Verification items for the finished model (mm, model axes). Give positions to 0.01 mm unless a question says otherwise; leave off trailing zeros. Order: outer loops, then holes, each group sorted by start corner. A loop starts at its lowest first (then second) coordinate and runs counter-clockwise, first axis right, second up. Notation, with made-up numbers: (-3.5, 82.25) - (40.5, 82.25) arc R21 ccw to (40.5, 87.25) - close; hole circle Ø4 at (46.25, 77). An arc over 180 degrees is marked (long way). Answer as a JSON object with one key per item and string values.
Autodesk Inventor part; units mm, degrees
ref_plane "YZ Plane" through (0, 0, 0) normal (1, 0, 0) x (0, 1, 0)
ref_plane "XZ Plane" through (0, 0, 0) normal (0, 1, 0) x (-1, 0, 0)
ref_plane "XY Plane" through (0, 0, 0) normal (0, 0, 1) x (1, 0, 0)
sketch "Sketch1" plane through (0, 0, 0) normal (0, 1, 0) x (-1, 0, 0)
  line L0 (0, 0) -> (12.7, 0)
  line L1 (0, 0) -> (0, -3.175)
  line L2 (12.7, 0) -> (12.7, -3.175)
  line L3 (12.7, -3.175) -> (0, -3.175)
  dimension "d2" = 3.175
  dimension "d3" = 12.7
extrude "Extrusion1" add sketch "Sketch1" along normal blind 209.55
sketch "Sketch2" plane through (-12.7, 0, 0) normal (0, 0, 1) x (1, 0, 0)
  line L0 (0, 209.55) -> (12.7, 209.55)
  line L1 (0, 0) -> (0, 209.55)
  line L2 (12.7, 0) -> (0, 0)
  point P0 (6.35, 201.93)
  point P1 (6.35, 50.8)
  dimension "d6" = 7.62
  dimension "d7" = 6.35
  dimension "d8" = 50.8
  dimension "d9" = 6.35
hole "Hole1" at (-6.35, 201.93, 0) at (-6.35, 50.8, 0) direction (0, 0, -1) diameter 6.35 end through all
properties part number "grabber articulation arms"
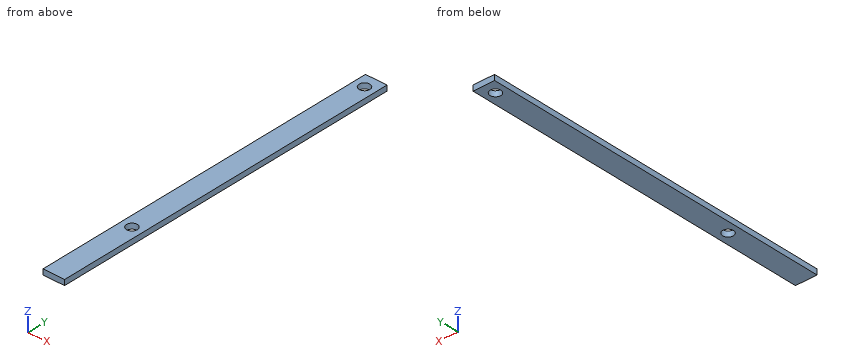
(1) Section check B-B (y = 50.8). Record the cut outline in (x, z) (3 decimals).
Computed values:
{"outline": "(-12.7, -3.175) - (-9.525, -3.175) - (-9.525, 0) - (-12.7, 0) - close; (-3.175, -3.175) - (0, -3.175) - (0, 0) - (-3.175, 0) - close"}
(2) Material ranges on line 1 along Y through (x, z) = (-6.5, -0.4); line 2 along X through (y, z) = (50.8, -2.5) (3 decimals); line 3 along Y through (x, z) = (-4.25, -0.3), recorded low to high. Write a range as [from, to].
Computed values:
{"line 1": "y = [0, 47.63], [53.97, 198.76], [205.1, 209.55]", "line 2": "x = [-12.7, -9.525], [-3.175, 0]", "line 3": "y = [0, 48.42], [53.18, 199.55], [204.31, 209.55]"}
(3) Section check A-A (x = -6.35). Record the cut outline in (y, z) (3 decimals).
Computed values:
{"outline": "(0, -3.175) - (47.625, -3.175) - (47.625, 0) - (0, 0) - close; (53.975, -3.175) - (198.755, -3.175) - (198.755, 0) - (53.975, 0) - close; (205.105, -3.175) - (209.55, -3.175) - (209.55, 0) - (205.105, 0) - close"}
(4) Section check C-C (z = -1.1). Record the cut outline in (x, y) (3 decimals), then the cut area to 3 significant figures.
Computed values:
{"outline": "(-12.7, 0) - (0, 0) - (0, 209.55) - (-12.7, 209.55) - close; hole circle Ø6.35 at (-6.35, 50.8); hole circle Ø6.35 at (-6.35, 201.93)", "area": "2,600 mm²"}
(5) Gauge pin test, flat end, axial feed: pin 1 Ø4 at (x, y) = (-6.35, 50.8) entering from -Z. Record the tip position at first contact, or that the pin passes through.
Computed values:
{"pin 1": "passes through"}
